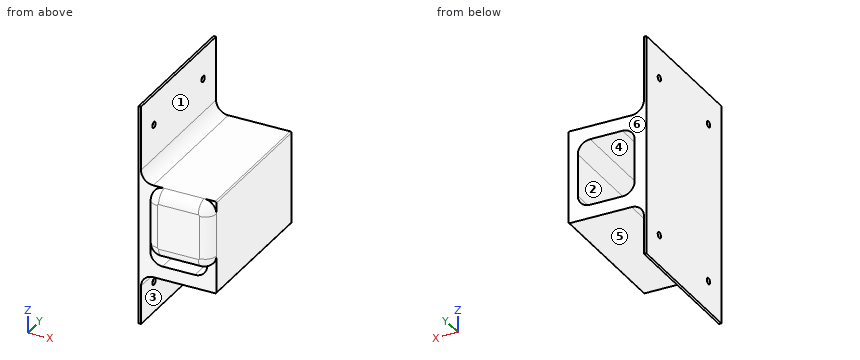
```python
from build123d import *

# Parameters (mm, degrees)
SKETCH1_W                       = 180
SKETCH1_H                       = 116
BOSS_EXTRUDE1_DEPTH             = 2
BOSS_EXTRUDE6_REACH             = 109.089
BOSS_EXTRUDE6_DIRECTION_2_REACH = 109.089
FILLET5_R                       = 10
BOSS_EXTRUDE8_DEPTH             = 8.98
FILLET7_R                       = 8.98
M6X1_0_TAPPED_HOLE1_D           = 5


with BuildPart() as part:
    # Sketch1 → Boss-Extrude1 (new body)
    with BuildSketch(Plane(origin=(0, 0, 0), x_dir=(0, 0, -1), z_dir=(1, 0, 0))):
        Rectangle(SKETCH1_W, SKETCH1_H)
    extrude(amount=BOSS_EXTRUDE1_DEPTH)

    # Boss-Extrude6: up to this face of the body (flat: up to its plane)
    boss_extrude6_end = Plane(part.part.faces().sort_by_distance((1, -58, 0))[0])
    # Sketch9 → Boss-Extrude6 (add, up to the picked face)
    with BuildSketch(Plane(origin=(0, 0, 0), x_dir=(1, 0, 0), z_dir=(0, 1, 0)), mode=Mode.PRIVATE) as boss_extrude6_sk1:
        with BuildLine():
            Line((2, -27.470907931), (20, -27.470907931))
            Line((20, -27.470907931), (62.451993428, -27.470907931))
            ThreePointArc((62.451993428, -27.470907931), (63.142907445, -27.184721975), (63.429093401, -26.493807958))
            Line((63.429093401, -26.493807958), (63.429093401, 47.609249241))
            ThreePointArc((63.429093401, 47.609249241), (63.142907445, 48.300163258), (62.451993428, 48.586349214))
            Line((62.451993428, 48.586349214), (20, 48.586349214))
            Line((20, 48.586349214), (2, 48.586349214))
            Line((2, 48.586349214), (2, 27.673016612))
            Line((2, 27.673016612), (2, -27.470907931))
        make_face()
        with BuildLine():
            Line((45.894546701, -16.622279359), (19.534546701, -16.622279359))
            ThreePointArc((19.534546701, -16.622279359), (12.463478889, -13.693347171), (9.534546701, -6.622279359))
            Line((9.534546701, -6.622279359), (9.534546701, 27.737720641))
            ThreePointArc((9.534546701, 27.737720641), (12.463478889, 34.808788453), (19.534546701, 37.737720641))
            Line((19.534546701, 37.737720641), (45.894546701, 37.737720641))
            ThreePointArc((45.894546701, 37.737720641), (52.965614513, 34.808788453), (55.894546701, 27.737720641))
            Line((55.894546701, 27.737720641), (55.894546701, -6.622279359))
            ThreePointArc((55.894546701, -6.622279359), (52.965614513, -13.693347171), (45.894546701, -16.622279359))
        make_face(mode=Mode.SUBTRACT)
    boss_extrude6_tool1 = split(extrude(boss_extrude6_sk1.sketch, amount=-BOSS_EXTRUDE6_REACH, mode=Mode.PRIVATE), bisect_by=boss_extrude6_end, keep=Keep.BOTH, mode=Mode.PRIVATE)
    add(boss_extrude6_tool1.solids().sort_by(Axis((11, 0, 26.493245), (0, -1, 0)))[0])

    # Boss-Extrude6 direction 2: up to this face of the body (flat: up to its plane)
    boss_extrude6_direction_2_end = Plane(part.part.faces().sort_by_distance((1, 58, 0))[0])
    # Sketch9 → Boss-Extrude6 direction 2 (add, up to the picked face)
    with BuildSketch(Plane(origin=(0, 0, 0), x_dir=(1, 0, 0), z_dir=(0, 1, 0)), mode=Mode.PRIVATE) as boss_extrude6_direction_2_sk1:
        with BuildLine():
            Line((2, -27.470907931), (20, -27.470907931))
            Line((20, -27.470907931), (62.451993428, -27.470907931))
            ThreePointArc((62.451993428, -27.470907931), (63.142907445, -27.184721975), (63.429093401, -26.493807958))
            Line((63.429093401, -26.493807958), (63.429093401, 47.609249241))
            ThreePointArc((63.429093401, 47.609249241), (63.142907445, 48.300163258), (62.451993428, 48.586349214))
            Line((62.451993428, 48.586349214), (20, 48.586349214))
            Line((20, 48.586349214), (2, 48.586349214))
            Line((2, 48.586349214), (2, 27.673016612))
            Line((2, 27.673016612), (2, -27.470907931))
        make_face()
        with BuildLine():
            Line((45.894546701, -16.622279359), (19.534546701, -16.622279359))
            ThreePointArc((19.534546701, -16.622279359), (12.463478889, -13.693347171), (9.534546701, -6.622279359))
            Line((9.534546701, -6.622279359), (9.534546701, 27.737720641))
            ThreePointArc((9.534546701, 27.737720641), (12.463478889, 34.808788453), (19.534546701, 37.737720641))
            Line((19.534546701, 37.737720641), (45.894546701, 37.737720641))
            ThreePointArc((45.894546701, 37.737720641), (52.965614513, 34.808788453), (55.894546701, 27.737720641))
            Line((55.894546701, 27.737720641), (55.894546701, -6.622279359))
            ThreePointArc((55.894546701, -6.622279359), (52.965614513, -13.693347171), (45.894546701, -16.622279359))
        make_face(mode=Mode.SUBTRACT)
    boss_extrude6_direction_2_tool1 = split(extrude(boss_extrude6_direction_2_sk1.sketch, amount=BOSS_EXTRUDE6_DIRECTION_2_REACH, mode=Mode.PRIVATE), bisect_by=boss_extrude6_direction_2_end, keep=Keep.BOTH, mode=Mode.PRIVATE)
    add(boss_extrude6_direction_2_tool1.solids().sort_by(Axis((11, 0, 26.493245), (0, 1, 0)))[0])

    # Fillet5
    fillet5_edges = [part.edges().sort_by_distance(p)[0] for p in [
        (2, 0, 27.470907931),
        (2, 0, -48.586349214),
    ]]
    fillet(fillet5_edges, radius=FILLET5_R)

    # Sketch11 → Boss-Extrude8 (add)
    with BuildSketch(Plane.XZ.offset(58)):
        with BuildLine():
            Line((21.022900027, -27.470907931), (53.429093401, -27.470907931))
            ThreePointArc((53.429093401, -27.470907931), (60.500161213, -24.541975743), (63.429093401, -17.470907931))
            Line((63.429093401, -17.470907931), (63.429093401, 17.470907931))
            ThreePointArc((63.429093401, 17.470907931), (60.500161213, 24.541975743), (53.429093401, 27.470907931))
            Line((53.429093401, 27.470907931), (21.022900027, 27.470907931))
            ThreePointArc((21.022900027, 27.470907931), (13.951832215, 24.541975743), (11.022900027, 17.470907931))
            Line((11.022900027, 17.470907931), (11.022900027, -17.470907931))
            ThreePointArc((11.022900027, -17.470907931), (13.951832215, -24.541975743), (21.022900027, -27.470907931))
        make_face()
    extrude(amount=BOSS_EXTRUDE8_DEPTH)

    # Fillet7
    fillet7_edges = [part.edges().sort_by_distance(p)[0] for p in [
        (60.500161213, -66.98, -24.541975743),
        (37.225996714, -66.98, -27.470907931),
        (13.951832215, -66.98, -24.541975743),
        (11.022900027, -66.98, 0),
        (13.951832215, -66.98, 24.541975743),
        (63.429093401, -66.98, 0),
        (60.500161213, -66.98, 24.541975743),
        (37.225996714, -66.98, 27.470907931),
    ]]
    fillet(fillet7_edges, radius=FILLET7_R - 0.0001)  # a hair under: the kernel refuses the full size

    # M6x1.0 Tapped Hole1 (through all)
    with Locations(Plane(origin=(2, 0, 0), x_dir=(0, 0, -1), z_dir=(1, 0, 0))):
        with Locations((-65, 38), (-65, -38), (65, -38), (65, 38)):
            Hole(M6X1_0_TAPPED_HOLE1_D / 2)


solid = part.part
```
Here's how the part is built. I have some questions about the finished solid (model axes, mm). Face numbers are marked on the shaded views. A direction names the side the tool comes from. Coordinates: 2 decimals unless noted, no trailing zeros. Order: outer loops, then holes, each group sorted by start corner. A loop starts at its lowest first (then second) coordinate and runs counter-clockwise, first axis right, second up.
1) Which directions (+Z, -Z, +X, -X, +Y, -Y) give clear straight access to the entire face, cutting with the end or side of a thin tool? Please do the marked faces 1, 2 and 3.
2) I need wall thicknesses on line 1 (Y direction, x = 1, z = -65); line 2 (Z direction, x = 46, y = 49); line 3 (X direction, y = -6.5, z = 52). Which ranges of each line are inside material? Lowest first, please.
3) Imagine slicing it at D-D on y = -10.5. List the corners of the cut face in (x, z) for me.
4) Will these pins go through, and if not, where does the flat tip stop? pin 1 (1.5 mm diameter, centred on x = 52.5, z = -33.5, fed in from -Y); pin 2 (12 mm diameter, centred on x = 17.5, z = -6, fed in from +Y); pin 3 (5 mm diameter, centred on x = 58.5, z = 21, fed in from -Y); pin 4 (3 mm diameter, centred on x = 38, y = -29.5, fed in from +Z).
5) We'd pull the mould along Z, two halves only. Please class the marked faces 4, 5 and 6: +Z half, -Z half, draft (parallel to the pull), parting line (faces both ways), or undercut.
6) Imagine slicing it at C-C on y = 38. List the corners of the cut face in (x, z) for me, and give its area (3 significant figures).
Response values:
1. face 1: +Z, +X, +Y, -Y
1. face 2: +Y
1. face 3: -Z, +X, +Y, -Y
2. line 1: y = -58 to -40.5, -35.5 to 35.5, 40.5 to 58
2. line 2: z = -48.59 to -37.74, 16.62 to 27.47
2. line 3: x = 0 to 2
3. outline: (0, -90) - (2, -90) - (2, -58.59) arc R10 cw to (12, -48.59) - (62.45, -48.59) arc R0.98 ccw to (63.43, -47.61) - (63.43, 26.49) arc R0.98 ccw to (62.45, 27.47) - (12, 27.47) arc R10 cw to (2, 37.47) - (2, 90) - (0, 90) - close; hole (9.53, -27.74) arc R10 ccw to (19.53, -37.74) - (45.89, -37.74) arc R10 ccw to (55.89, -27.74) - (55.89, 6.62) arc R10 ccw to (45.89, 16.62) - (19.53, 16.62) arc R10 ccw to (9.53, 6.62) - close
4. pin 1: passes through
4. pin 2: stops at y = -58
4. pin 3: stops at y = -66.58
4. pin 4: stops at z = 27.47
5. face 4: undercut
5. face 5: -Z half
5. face 6: draft
6. outline: (0, -90) - (2, -90) - (2, -67.5) - (0, -67.5) - close; (0, -62.5) - (2, -62.5) - (2, -58.59) arc R10 cw to (12, -48.59) - (62.45, -48.59) arc R0.98 ccw to (63.43, -47.61) - (63.43, 26.49) arc R0.98 ccw to (62.45, 27.47) - (12, 27.47) arc R10 cw to (2, 37.47) - (2, 62.5) - (0, 62.5) - close; (0, 67.5) - (2, 67.5) - (2, 90) - (0, 90) - close; hole (9.53, -27.74) arc R10 ccw to (19.53, -37.74) - (45.89, -37.74) arc R10 ccw to (55.89, -27.74) - (55.89, 6.62) arc R10 ccw to (45.89, 16.62) - (19.53, 16.62) arc R10 ccw to (9.53, 6.62) - close
6. area: 2,620 mm2
